The listing builds one solid part. Answer for the finished solid, in the listing's coordinates (mm). A direction names the side the tool comes from. Coordinates: 2 decimals unless noted, no trailing zeros. Order: outer loops, then holes, each group sorted by start corner. A loop starts at its lowest first (then second) coordinate and runs counter-clockwise, first axis right, second up. Notation, with made-up numbers: (-33, 45) -> (7, 45) arc R6 ccw to (7, 50) -> close; hole circle Ø6 at (22.25, -31.75). An arc over 180 degrees is marked (long way). Answer in a Markdown table with one row per item. Add a question column.
```python
from build123d import *

# Parameters (mm, degrees)
SM_BASE_FLANGE_1_DEPTH           = 3
SKETCH_6_R                       = 2.5
CUT_EXTRUDE_1_DEPTH              = 3
CUT_EXTRUDE_2_REACH              = 68.106
SKETCH_9_R                       = 11
HOLE_WIZARD_M3_1_D               = 2.5
HOLE_WIZARD_M3_1_DEPTH           = 7.5
HOLE_WIZARD_M3_1_TIP             = 0.751075774
SM_EDGE_FLANGE_1_STRIP_W         = 13.4732
SM_EDGE_FLANGE_1_STRIP_H         = 3
SM_EDGE_FLANGE_1_STRIP_CUT_DEPTH = 32
SM_EDGE_FLANGE_1_DEPTH           = 32
HOLE_WIZARD_7_0_7_D              = 7
HOLE_WIZARD_7_0_7_DEPTH          = 6
HOLE_WIZARD_7_0_7_TIP            = 2.103012167
FILLET_1_R                       = 5
CHAMFER_1_SIZE                   = 1
HOLE_WIZARD_4_5_4_5_1_D          = 4.5
HOLE_WIZARD_4_5_4_5_1_DEPTH      = 5
HOLE_WIZARD_4_5_4_5_1_TIP        = 1.351936393
HOLE_WIZARD_M4_1_D               = 3.3
HOLE_WIZARD_M4_1_DEPTH           = 11.5
HOLE_WIZARD_M4_1_TIP             = 0.991420021


# Sheet-metal steps are written as plain solids
with BuildPart() as part:
    # Sketch 1 → 基体-法兰1 (new body)
    with BuildSketch(Plane.XY):
        Polygon((20, -25), (16, -25), (16, -35), (-16, -35), (-16, -25), (-56, -25), (-56, 6), (-25, 6), (-25, 26.339745962), (-20, 35), (20, 35), (25, 26.339745962), (25, -20), align=None)
    extrude(amount=-SM_BASE_FLANGE_1_DEPTH)

    # Sketch 6 → 切除-拉伸1 (cut)
    with BuildSketch(Plane.XY):
        with Locations((-17.8, -5)):
            Circle(SKETCH_6_R)
        with Locations((17.8, -5)):
            Circle(SKETCH_6_R)
        with Locations((0, 29)):
            Circle(SKETCH_6_R)
        with Locations((-12.5, 25)):
            Circle(SKETCH_6_R)
        with Locations(Location((12.5, 25, 0), (0, 0, 180))):
            Circle(SKETCH_6_R)
    extrude(amount=-CUT_EXTRUDE_1_DEPTH, mode=Mode.SUBTRACT)

    # Sketch 9 → 切除-拉伸2 (cut, up to next)
    with BuildSketch(Plane(origin=(0, 0, -3), x_dir=(-1, 0, 0), z_dir=(0, 0, -1)), mode=Mode.PRIVATE) as cut_extrude_2_sk1:
        with Locations((17.8, -5)):
            Circle(SKETCH_9_R)
    cut_extrude_2_tool1 = extrude(cut_extrude_2_sk1.sketch, amount=-CUT_EXTRUDE_2_REACH, mode=Mode.PRIVATE) & part.part
    add(cut_extrude_2_tool1.solids().sort_by_distance((-17.8, -5, -3))[0], mode=Mode.SUBTRACT)

    # M3 螺纹孔1
    with Locations(Plane(origin=(0, -38, 0), x_dir=(-1, 0, 0), z_dir=(0, 0, 1))):
        with Locations((51.965, -38), (51.965, -28), (3.335, -28), (3.335, -38)):
            Hole(HOLE_WIZARD_M3_1_D / 2, depth=HOLE_WIZARD_M3_1_DEPTH)
            with Locations((0, 0, -(HOLE_WIZARD_M3_1_DEPTH + HOLE_WIZARD_M3_1_TIP / 2))):  # 118° drill point
                Cone(0, HOLE_WIZARD_M3_1_D / 2, HOLE_WIZARD_M3_1_TIP, mode=Mode.SUBTRACT)

    # 边线-法兰1 strip (across the edge) → 边线-法兰1 strip cut (cut)
    with BuildSketch(Plane(origin=(16, -35, -3), x_dir=(0, 1, 0), z_dir=(-1, 0, 0))):
        with Locations((-6, -1.5)):
            Rectangle(SM_EDGE_FLANGE_1_STRIP_W, SM_EDGE_FLANGE_1_STRIP_H)
    extrude(amount=SM_EDGE_FLANGE_1_STRIP_CUT_DEPTH, mode=Mode.SUBTRACT)

    # 边线-法兰1 section (across the edge) → 边线-法兰1 (add)
    with BuildSketch(Plane(origin=(16, -35, -3), x_dir=(0, 1, 0), z_dir=(-1, 0, 0))):
        with BuildLine():
            Line((-3, 0.7366), (-3, 18))
            Line((-3, 18), (0, 18))
            Line((0, 18), (0, 0.7366))
            ThreePointArc((0, 0.7366), (0.215745145, 0.215745145), (0.7366, 0))
            Line((0.7366, 0), (0.7366, -3))
            ThreePointArc((0.7366, -3), (-1.905575199, -1.905575199), (-3, 0.7366))
        make_face()
    extrude(amount=SM_EDGE_FLANGE_1_DEPTH)

    # Ø7.0 (7) 直径孔
    with Locations(Plane(origin=(-9.85, -35, 1.271), x_dir=(1, 0, 0), z_dir=(0, 1, 0))):
        with Locations((9.85, 9.75)):
            Hole(HOLE_WIZARD_7_0_7_D / 2, depth=HOLE_WIZARD_7_0_7_DEPTH)
            with Locations((0, 0, -(HOLE_WIZARD_7_0_7_DEPTH + HOLE_WIZARD_7_0_7_TIP / 2))):  # 118° drill point
                Cone(0, HOLE_WIZARD_7_0_7_D / 2, HOLE_WIZARD_7_0_7_TIP, mode=Mode.SUBTRACT)

    # 圆角1
    fillet_1_edges = [part.edges().sort_by_distance(p)[0] for p in [
        (-25, 6, -1.5),
    ]]
    fillet(fillet_1_edges, radius=FILLET_1_R)

    # 倒角1
    chamfer_1_edges = [part.edges().sort_by_distance(p)[0] for p in [
        (-56, -25, -1.5),
        (-56, 6, -1.5),
    ]]
    chamfer(chamfer_1_edges, length=CHAMFER_1_SIZE)

    # Ø4.5 (4.5) 直径孔1
    with Locations(Plane(origin=(-9.85, -35, 1.271), x_dir=(1, 0, 0), z_dir=(0, 1, 0))):
        with Locations((-1.15, 17.75), (20.85, 17.75)):
            Hole(HOLE_WIZARD_4_5_4_5_1_D / 2, depth=HOLE_WIZARD_4_5_4_5_1_DEPTH)
            with Locations((0, 0, -(HOLE_WIZARD_4_5_4_5_1_DEPTH + HOLE_WIZARD_4_5_4_5_1_TIP / 2))):  # 118° drill point
                Cone(0, HOLE_WIZARD_4_5_4_5_1_D / 2, HOLE_WIZARD_4_5_4_5_1_TIP, mode=Mode.SUBTRACT)

    # M4 螺纹孔1
    with Locations(Plane(origin=(-9.85, -49.5, 0), x_dir=(-1, 0, 0), z_dir=(0, 0, 1))):
        with Locations((-2.35, -24.5), (-17.35, -24.5)):
            Hole(HOLE_WIZARD_M4_1_D / 2, depth=HOLE_WIZARD_M4_1_DEPTH)
            with Locations((0, 0, -(HOLE_WIZARD_M4_1_DEPTH + HOLE_WIZARD_M4_1_TIP / 2))):  # 118° drill point
                Cone(0, HOLE_WIZARD_M4_1_D / 2, HOLE_WIZARD_M4_1_TIP, mode=Mode.SUBTRACT)


solid = part.part
```
Q1. For faces 4 (the face through (-6, 1, -3)), 5 (the face through (-16, -35.3, -7.4)), 6 (the face through (-43, 6, -1)), determine the directions among +Z, -Z, +X, -X, +Y, -Y from which every point of the face is accessible in a straight line to the end or side of a thin tool.
Q2. A cutting plane is placed at C-C (x = -11). Determine the outline of the cut face in (y, z).
Q3. A cutting plane is placed at B-B (y = 25). Determine the outline of the cut face in (x, z).
Q4. A cutting plane is placed at D-D (z = -7). Determine the outline of the cut face in (x, y).
Q5. Straight lines are drawn through the part: line 1 (Y direction, x = -12.5, z = -2.25); line 2 (X direction, y = -10, z = -1.3) (3 decimals); line 3 (Y direction, x = -7, z = -6.25). For each, find the intervals that lie inside material, in ascending order.
Q6. A cutting plane is placed at A-A (x = 17.8). Determine the outline of the cut face in (y, z).
Q7. Determine the mould class of faces 1 (the face through (-2.66, -11.05, -1.52)), 2 (the face through (0, -37, -21)), 3 (the face through (18, -25, -1)) for opening direction Y: +Y half, -Y half, draft (parallel to the pull), parting line (faces both ways), or undercut.
Q8. Given pin 1 (3 mm diameter, centred on x = -3.335, y = -10, fed in from -Z); pin 2 (6.5 mm diameter, centred on y = -33.5, z = -7.5, fed in from -X); pin 3 (3.5 mm diameter, centred on x = 18.5, z = -1, fed in from -Y), each flat-ended and moving along its own axis, determine where each tip first touches the part or whether it passes through.
Returned:
| question | item | result |
|---|---|---|
| 1 | face 4 | -Z, +X, -X, +Y |
| 1 | face 5 | +Z, -Z, -X, -Y |
| 1 | face 6 | +Z, -Z, -X, +Y |
| 2 | outline | (-38, -21) -> (-35, -21) -> (-35, -18.73) -> (-38, -18.73) -> close; (-38, -14.23) -> (-35, -14.23) -> (-35, -3.74) arc R0.74 cw to (-34.26, -3) -> (-13.65, -3) -> (-13.65, 0) -> (-34.26, 0) arc R3.74 ccw to (-38, -3.74) -> close; (3.65, -3) -> (23, -3) -> (23, 0) -> (3.65, 0) -> close; (27, -3) -> (35, -3) -> (35, 0) -> (27, 0) -> close |
| 3 | outline | (-25, -3) -> (-15, -3) -> (-15, 0) -> (-25, 0) -> close; (-10, -3) -> (10, -3) -> (10, 0) -> (-10, 0) -> close; (15, -3) -> (25, -3) -> (25, 0) -> (15, 0) -> close |
| 4 | outline | (-16, -38) -> (-3.17, -38) -> (-3.17, -35) -> (-16, -35) -> close; (3.17, -38) -> (16, -38) -> (16, -35) -> (3.17, -35) -> close |
| 5 | line 1 | y = -37.69 to -14.64, 4.64 to 22.5, 27.5 to 35 |
| 5 | line 2 | x = -56 to -53.215, -50.715 to -27.598, -8.002 to -4.585, -2.085 to 25 |
| 5 | line 3 | y = -38 to -35 |
| 6 | outline | (-25, -3) -> (-7.5, -3) -> (-7.5, 0) -> (-25, 0) -> close; (-2.5, -3) -> (35, -3) -> (35, 0) -> (-2.5, 0) -> close |
| 7 | face 1 | undercut |
| 7 | face 2 | draft |
| 7 | face 3 | -Y half |
| 8 | pin 1 | stops at z = -3 |
| 8 | pin 2 | stops at x = -16 |
| 8 | pin 3 | stops at y = -25 |
